Geometry check sheet. Reference: the model listing, model coordinates, mm. Give positions to 0.01 mm unless a question says otherwise; leave off trailing zeros. Loops run counter-clockwise (first coordinate to the right, second up) from the corner with the lowest first, then second, coordinate; pieces in that order, holes last.
1. Cross-section at C-C, the plane x = 0. Record the cut outline in (y, z).
2. Cross-section at B-B, the plane z = 0. Record the cut outline in (x, y), plus the area to 3 significant figures.
3. Go/stop test with flat-tipped pins: pin 1 Ø2.5 at (y, z) = (3.5, 11) entering from +X; pin 2 Ø1.5 at (y, z) = (2, 52.5) entering from +X. Record where each tip stops, or that it passes through.
4. Cross-section at D-D, the plane x = -12.25. Record the cut outline in (y, z).
5. Cross-section at A-A, the plane y = 4.2. Record the cut outline in (x, z).
6. Material ranges on L1, parallel to X at y = 0.65, z = 0; L2, parallel to Z at x = -4, y = 4.7; L3, parallel to X at y = 3.95, z = 10, recorded low to high.
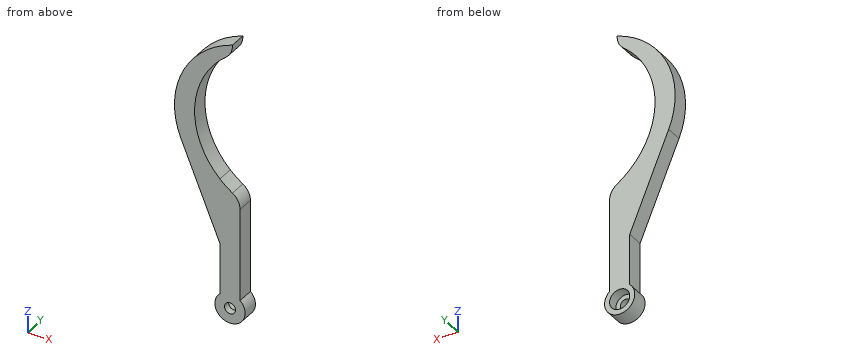
from build123d import *

# Parameters (mm, degrees)
EXTRUDE_2_DEPTH     = 5
SKETCH_4_R          = 1.65
CUT_EXTRUDE_1_DEPTH = 5
EXTRUDE_3_DEPTH     = 5
SKETCH_7_R          = 3
CUT_EXTRUDE_2_DEPTH = 3
CUT_EXTRUDE_3_DEPTH = 7.5
EXTRUDE_4_DEPTH     = 5
FILLET_1_R          = 5


with BuildPart() as part:
    # 草图3 → 凸台-拉伸2 (new body)
    with BuildSketch(Plane(origin=(0, 0, 0), x_dir=(1, 0, 0), z_dir=(0, 1, 0))):
        with BuildLine():
            Line((-3, -3.354101966), (-3, -7.416198487))
            Line((-3, -7.416198487), (-3, -43.854101966))
            Line((-3, -43.854101966), (3, -43.854101966))
            Line((3, -43.854101966), (3, -10.583005244))
            Line((3, -10.583005244), (3, -7.416198487))
            Line((3, -7.416198487), (3, -3.354101966))
            ThreePointArc((3, -3.354101966), (0, 4.5), (-3, -3.354101966))
        make_face()
    extrude(amount=EXTRUDE_2_DEPTH)

    # 草图4 → 切除-拉伸1 (cut)
    with BuildSketch(Plane(origin=(0, 5, 0), x_dir=(1, 0, 0), z_dir=(0, 1, 0))):
        with Locations(Location((0, 0, 0), (0, 0, 270))):
            Circle(SKETCH_4_R)
    extrude(amount=-CUT_EXTRUDE_1_DEPTH, mode=Mode.SUBTRACT)

    # 草图6 → 凸台-拉伸3 (add)
    with BuildSketch(Plane(origin=(0, 5, 0), x_dir=(1, 0, 0), z_dir=(0, 1, 0))):
        with BuildLine():
            Line((3, -33.74604712), (-3, -33.74604712))
            ThreePointArc((-3, -33.74604712), (-16.46902092, -57.986607816), (0.722500961, -79.745993902))
            Line((0.722500961, -79.745993902), (1.949520222, -77.620734201))
            ThreePointArc((1.949520222, -77.620734201), (-10.543317179, -55.371702353), (3, -33.74604712))
        make_face()
    extrude(amount=-EXTRUDE_3_DEPTH)

    # 草图7 → 切除-拉伸2 (cut)
    with BuildSketch(Plane(origin=(0, 5, 0), x_dir=(1, 0, 0), z_dir=(0, 1, 0))):
        with Locations(Location((0, 0, 0), (0, 0, 270))):
            Circle(SKETCH_7_R)
    extrude(amount=-CUT_EXTRUDE_2_DEPTH, mode=Mode.SUBTRACT)

    # 草图8 → 切除-拉伸3 (cut)
    with BuildSketch(Plane(origin=(0, 5, 0), x_dir=(1, 0, 0), z_dir=(0, 1, 0))):
        with BuildLine():
            Line((-3, -38.067187498), (-3, -43.854101966))
            Line((-3, -43.854101966), (3, -43.854101966))
            Line((3, -43.854101966), (3, -33.74604712))
            ThreePointArc((3, -33.74604712), (-0.160637142, -35.683569047), (-3, -38.067187498))
        make_face()
    extrude(amount=-CUT_EXTRUDE_3_DEPTH, mode=Mode.SUBTRACT)

    # 草图9 → 凸台-拉伸4 (add)
    with BuildSketch(Plane(origin=(0, 5, 0), x_dir=(1, 0, 0), z_dir=(0, 1, 0))):
        with BuildLine():
            Line((-3, -18.550074543), (-14.614967684, -46.324924269))
            ThreePointArc((-14.614967684, -46.324924269), (-9.917875534, -39.010182445), (-3, -33.74604712))
            Line((-3, -33.74604712), (-3, -18.550074543))
        make_face()
    extrude(amount=-EXTRUDE_4_DEPTH)

    # 圆角1
    # the kernel refuses this fillet: 5 mm, written as the material it takes off along each edge
    with BuildSketch(Plane(origin=(1.949520222, 14.371610933, 77.620734201), x_dir=(-0.4999999999999996, 0, 0.8660254037844388), z_dir=(0, -1, 0))) as fillet_1_piece_1:
        with BuildLine():
            CenterArc((4.662743969, 4.485712903), FILLET_1_R, 188.59932897, 55.185648669)
            Line((-0.281046693, 3.738094086), (-0.379922506, 3.723141709))
            ThreePointArc((-0.379922506, 3.723141709), (-0.170079243, 1.866824898), (-0.1, 0))
            Line((-0.1, 0), (0, -0.1))
            ThreePointArc((0, -0.1), (1.227019261, -0.1), (2.409864412, -0.089714258))
            Line((2.409864412, -0.089714258), (2.454038521, 0))
        make_face()
    extrude(amount=23.743221866, mode=Mode.SUBTRACT)
    with BuildSketch(Plane(origin=(3, 12.160146085, 33.74604712), x_dir=(0, 0, -1), z_dir=(0, -1, 0))) as fillet_1_piece_2:
        with BuildLine():
            CenterArc((2.864058434, -5), FILLET_1_R, 90, 56.748348073)
            Line((-1.317293303, -2.258413296), (-1.400920337, -2.203581562))
            ThreePointArc((-1.400920337, -2.203581562), (-0.715482953, -1.096055019), (-0.088896208, 0.045798081))
            Line((-0.088896208, 0.045798081), (0, 0.1))
            Line((0, 0.1), (2.864058434, 0.1))
            Line((2.864058434, 0.1), (2.864058434, 0))
        make_face()
    extrude(amount=19.320292171, mode=Mode.SUBTRACT)


solid = part.part
Result:
1. outline: (0, -4.5) - (5, -4.5) - (5, -3) - (2, -3) - (2, -1.65) - (0, -1.65) - close; (0, 1.65) - (2, 1.65) - (2, 3) - (5, 3) - (5, 35.57) - (0, 35.57) - close; (0, 76.81) - (5, 76.81) - (5, 79.5) - (0, 79.5) - close
2. outline: (-4.5, 0) - (-1.65, 0) - (-1.65, 2) - (-3, 2) - (-3, 5) - (-4.5, 5) - close; (1.65, 0) - (4.5, 0) - (4.5, 5) - (3, 5) - (3, 2) - (1.65, 2) - close
2. area: 20.4 mm2
3. pin 1: stops at x = 3
3. pin 2: stops at x = -10.19
4. outline: (0, 40.67) - (5, 40.67) - (5, 69.99) - (0, 69.99) - close
5. outline: (-14.61, 46.32) - (-3, 18.55) - (-3, 3.35) arc R4.5 ccw (long way) to (3, 3.35) - (3, 30.88) arc R5 ccw to (0.74, 35.06) arc R25 cw to (-1.15, 75.51) arc R5 ccw to (0.72, 79.75) arc R25 ccw to start; hole circle Ø6 at (0, 0)
6. L1: x = -4.5 to -1.65, 1.65 to 4.5
6. L2: z = -2.06 to 2.06, 20.94 to 39.1, 72.84 to 77.65
6. L3: x = -3 to 3
